Input: part model. Units: mm. Frame: model coordinates. A direction names the side the tool comes from. Coordinates: 2 decimals unless noted, no trailing zeros. Order: outer loops, then holes, each group sorted by start corner. A loop starts at its lowest first (then second) coordinate and runs counter-clockwise, first axis right, second up. Notation, with made-up numbers: (28, 51.5) -> (36, 51.5) arc R21 ccw to (36, 57.5) -> close; hole circle Ø2 at (37, -19). An arc over 180 degrees is marked (long way). Write each question's results on one line, items separated by ' | '.
```python
from build123d import *

# Parameters (mm, degrees)
F3_DEPTH = 150
F6_DEPTH = 227.39467
F7_DEPTH = 227.39467


with BuildPart() as f3:
    # F2 (on line) → F3 (new body)
    with BuildSketch(Plane.YZ.offset(263.697335)):
        Polygon((0, 320), (0, 0), (92.3760430703, 0), (184.7520861407, 160), (92.3760430703, 320), align=None)
        Polygon((-92.3760430703, 0), (0, 0), (0, 320), (-92.3760430703, 320), (-184.7520861407, 160), align=None)
    extrude(amount=-F3_DEPTH)


with BuildPart() as f4_1:
    # F4: instance of F3
    add(f3.part.mirror(Plane.YZ))


with BuildPart() as f3_1:
    add(f3.part)

    add(f4_1.part)  # F6 merges F4_1
    # F5 (on face) → F6 (join, through all)
    with BuildSketch(Plane(origin=(113.697335, 0, 0), x_dir=(0, -1, 0), z_dir=(-1, 0, 0))):
        Polygon((-149.9936365076, 99.7965992432), (-92.3760430703, 0), (-34.7584496331, 99.7965992432), align=None)
        with BuildLine():
            Line((-34.7584496331, 99.7965992432), (-92.3760430703, 0))
            Line((-92.3760430703, 0), (92.3760430703, 0))
            Line((92.3760430703, 0), (34.7584496331, 99.7965992432))
            Line((34.7584496331, 99.7965992432), (20.8100413197, 99.7965992432))
            ThreePointArc((20.8100413197, 99.7965992432), (0, 97.6046816163), (-20.8100413197, 99.7965992432))
            Line((-20.8100413197, 99.7965992432), (-34.7584496331, 99.7965992432))
        make_face()
        Polygon((34.7584496331, 99.7965992432), (92.3760430703, 0), (149.9936365076, 99.7965992432), align=None)
    extrude(amount=F6_DEPTH)

    # F5 (on face) → F7 (join, through all)
    with BuildSketch(Plane(origin=(113.697335, 0, 0), x_dir=(0, -1, 0), z_dir=(-1, 0, 0))):
        with BuildLine():
            Line((-92.5799725491, 160), (0, 160))
            Line((0, 160), (0, 297.366897697))
            ThreePointArc((0, 297.366897697), (-82.8261973956, 253.3074410864), (-92.5799725491, 160))
        make_face()
        with BuildLine():
            Line((0, 297.366897697), (0, 160))
            Line((0, 160), (65.2852114178, 273.0773031585))
            ThreePointArc((65.2852114178, 273.0773031585), (34.8286636002, 291.0977543577), (0, 297.366897697))
        make_face()
        with BuildLine():
            Line((65.2852114178, 273.0773031585), (0, 160))
            Line((0, 160), (92.5799725491, 160))
            ThreePointArc((92.5799725491, 160), (98.0388341014, 178.3906920813), (99.8811080403, 197.4857896566))
            ThreePointArc((99.8811080403, 197.4857896566), (90.8212392517, 239.0518604856), (65.2852114178, 273.0773031585))
        make_face()
        with BuildLine():
            Line((92.5799725491, 160), (0, 160))
            Line((0, 160), (32.8215652942, 103.1513813265))
            ThreePointArc((32.8215652942, 103.1513813265), (68.8427758348, 125.1193059869), (92.5799725491, 160))
        make_face()
        with BuildLine():
            ThreePointArc((-92.5799725491, 160), (-68.8427758348, 125.1193059868), (-32.8215652942, 103.1513813265))
            Line((-32.8215652942, 103.1513813265), (0, 160))
            Line((0, 160), (-92.5799725491, 160))
        make_face()
    extrude(amount=F7_DEPTH)


solid = f3_1.part
```
(1) Cut plane B-B, the plane y = -138.5. Return loops of the section in (x, z).
Return value:
outline: (-263.7, 79.89) -> (263.7, 79.89) -> (263.7, 240.11) -> (113.7, 240.11) -> (113.7, 99.8) -> (-113.7, 99.8) -> (-113.7, 240.11) -> (-263.7, 240.11) -> close
(2) Cut plane C-C, the plane x = 156.5. Return loops of the section in (y, z), plus the area to 3 significant figures.
Return value:
outline: (-184.75, 160) -> (-92.38, 0) -> (92.38, 0) -> (184.75, 160) -> (92.38, 320) -> (-92.38, 320) -> close | area: 88,700 mm2
(3) Line query: line 1 along X through (y, z) = (-114, 100); line 2 along Y through (x, z) = (-29, 111.5); line 3 along Z through (x, y) = (-12.5, -74.5). Output: solid intervals per line, ascending. Write a range as from..to.
Return value:
line 1: -263.7..-113.7, 113.7..263.7 | line 2: -50.82..-28, 28..50.82 | line 3: 0..99.8, 130.96..264.01
(4) Cut plane A-A, the plane x = -80. Return loops of the section in (y, z), plus the area to 3 significant figures.
Return value:
outline: (-149.99, 99.8) -> (-92.38, 0) -> (92.38, 0) -> (149.99, 99.8) -> (20.81, 99.8) arc R99.88 cw to (-20.81, 99.8) -> close; (-32.82, 103.15) -> (0, 160) -> (32.82, 103.15) arc R99.88 ccw (long way) to start | area: 53,400 mm2
(5) Cut plane D-D, the plane z = 230. Return loops of the section in (x, y).
Return value:
outline: (-263.7, -144.34) -> (-113.7, -144.34) -> (-113.7, -94.44) -> (113.7, -94.44) -> (113.7, -144.34) -> (263.7, -144.34) -> (263.7, 144.34) -> (113.7, 144.34) -> (113.7, 94.44) -> (-113.7, 94.44) -> (-113.7, 144.34) -> (-263.7, 144.34) -> close
(6) Reachability of faces 1 (the face through (113.697, -3, 136)), 2 (the face through (2, 84, 99.797)), 3 (the face through (-263.697, -3, 162)) from +Z, -Z, +X, -X, +Y, -Y: full face, straight path, thin tool, end or side. Return the list, or none.
Return value:
face 1: none | face 2: +Y, -Y | face 3: +Z, -Z, -X, +Y, -Y
(7) Mould query, pull axis Z, two halves, no side actions, for faces 4 (the face through (189.747, -137.917, 241.12)), 5 (the face through (1.592, -0.293, 97.605)), 6 (the face through (263.697, -3, 162)), 7 (the face through (2, -86, 99.797)). Classes: +Z half, -Z half, draft (parallel to the pull), parting line (faces both ways), or undercut.
Return value:
face 4: +Z half | face 5: undercut | face 6: draft | face 7: undercut
(8) Pin query (flat end, axial travel): P1, Ø1, axis at x = 100, y = -92, coming from the -Z side; P2, Ø1, axis at x = 12, y = -103, coming from the -Z side; P3, Ø4, axis at x = -114, z = 145, coming from the +Y side; P4, Ø1.5, axis at x = -206.5, z = 34.5, coming from the +Y side. Return the tip coordinate at first contact, or that it passes through.
Return value:
P1: z = 0 | P2: z = 17.54 | P3: y = 177.25 | P4: y = 112.73
